CAD build for the part. Positions are in the model's coordinates, mm. A direction names the side the tool comes from. Coordinates: 2 decimals unless noted, no trailing zeros. Loops run counter-clockwise (first coordinate to the right, second up) from the corner with the lowest first, then second, coordinate; pieces in that order, holes last. Notation, with made-up numbers: (65, 58) -> (110, 58) arc R25 cw to (110, 77) -> close; hole circle Ø2 at (1.5, 68.5). An arc over 180 degrees is marked (long way). Write item = value, one per line. Start each with the question number.
(1) Tool access for faces 1 (the face through (2.958, -2.562, -32.586)), 2 (the face through (1.479, -11.495, -26.118)): list every direction of +Z, -Z, +X, -X, +Y, -Y with a clear straight run to the whole face (end or side of a thin tool).
(2) Pull direction Y, two halves, no side cores. Call faces 3 (the face through (2.96, -1.92, -10.54)), 4 (the face through (4.479, 12.156, -18.385)), 5 (the face through (4.48, -12.82, -17.36)), 6 (the face through (0, -3, -21)): +Y half, -Y half, draft (parallel to the pull), parting line (faces both ways), or undercut.
(3) Band-saw the part on C-C (x = 1.9). Write the cut outline in (y, z).
(4) Flat gauge pins, fed straight in: P1, Ø6, axis at y = -12.99, z = -21.36, coming from the +X side; P2, Ø3.5, axis at y = 12, z = -13.43, coming from the -X side; P3, Ø2, axis at x = 4, y = 0.5, coming from the -Z side. Where does each tip first touch, or does it go through?
(5) Band-saw the part on A-A (y = 12). Write the cut outline in (x, z), and give its area (3 significant figures).
(6) Drill centre lines: line 1 (Z direction, x = 3.95, y = 12); line 2 (Y direction, x = 5.55, z = -23.75); line 3 (Z direction, x = 1.25, y = -14.5). Where is each one in solid material? Low to high. Write a range as from..to.
(7) Band-saw the part on D-D (y = -10). Write the cut outline in (x, z), and give its area (3 significant figures).
(8) Band-saw the part on B-B (z = -24). Write the cut outline in (x, y), and give its area (3 significant figures).
```python
from build123d import *

# Parameters (mm, degrees)
SKETCH1_R           = 3.55
SKETCH1_R_2         = 1.5
SKETCH1_R_3         = 4
BOSS_EXTRUDE1_DEPTH = 6
SKETCH2_R           = 4.99
CUT_EXTRUDE1_DEPTH  = 3
SKETCH3_R           = 12.55
CUT_EXTRUDE2_DEPTH  = 3


with BuildPart() as part:
    # Sketch1 → Boss-Extrude1 (new body)
    with BuildSketch(Plane(origin=(0, 0, 0), x_dir=(0, 0, -1), z_dir=(1, 0, 0))):
        with BuildLine():
            Line((30.431712199, 18), (13.431712199, 18))
            ThreePointArc((13.431712199, 18), (8.728856289, 15.726009432), (7.590750373, 10.627715428))
            Line((7.590750373, 10.627715428), (13.570211844, -14.823132675))
            ThreePointArc((13.570211844, -14.823132675), (21.189386747, -20.991639419), (29.061992727, -15.150032042))
            Line((29.061992727, -15.150032042), (36.209586036, 10.382540903))
            ThreePointArc((36.209586036, 10.382540903), (35.212128216, 15.625965073), (30.431712199, 18))
        make_face()
        with Locations((21.931712199, 12)):
            Circle(SKETCH1_R, mode=Mode.SUBTRACT)
        with Locations((30.431712199, 12)):
            Circle(SKETCH1_R_2, mode=Mode.SUBTRACT)
        with Locations((13.431712199, 12)):
            Circle(SKETCH1_R_2, mode=Mode.SUBTRACT)
        with Locations((21.358160945, -12.993419913)):
            Circle(SKETCH1_R_3, mode=Mode.SUBTRACT)
    extrude(amount=BOSS_EXTRUDE1_DEPTH)

    # Sketch2 → Cut-Extrude1 (cut)
    with BuildSketch(Plane(origin=(0, 0, 0), x_dir=(0, 0, -1), z_dir=(1, 0, 0))):
        with Locations((21.358160945, -12.993419913)):
            Circle(SKETCH2_R)
    extrude(amount=CUT_EXTRUDE1_DEPTH, mode=Mode.SUBTRACT)

    # Sketch3 → Cut-Extrude2 (cut)
    with BuildSketch(Plane(origin=(0, 0, 0), x_dir=(0, 0, -1), z_dir=(1, 0, 0))):
        with Locations((21.931712199, 12)):
            Circle(SKETCH3_R)
    extrude(amount=CUT_EXTRUDE2_DEPTH, mode=Mode.SUBTRACT)


solid = part.part
```
Findings below:
q1.face_1 = -Z, +X, -X, -Y
q1.face_2 = -X
q2.face_3 = -Y half
q2.face_4 = undercut
q2.face_5 = undercut
q2.face_6 = draft
q3.outline = (-15.15, -29.06) -> (10.38, -36.21) arc R6 ccw to (17.25, -33.33) arc R12.55 cw (long way) to (17.25, -10.53) arc R6 ccw to (10.63, -7.59) -> (-14.82, -13.57) arc R8 ccw to start; hole circle Ø9.98 at (-12.99, -21.36)
q4.P1 = through
q4.P2 = 3
q4.P3 = -33.72
q5.outline = (0, -36.43) -> (6, -36.43) -> (6, -31.93) -> (3, -31.93) -> (3, -34.48) -> (0, -34.48) -> close; (0, -9.38) -> (3, -9.38) -> (3, -11.93) -> (6, -11.93) -> (6, -7.43) -> (0, -7.43) -> close; (3, -28.93) -> (6, -28.93) -> (6, -25.48) -> (3, -25.48) -> close; (3, -18.38) -> (6, -18.38) -> (6, -14.93) -> (3, -14.93) -> close
q5.area = 59.4 mm²
q6.line_1 = -36.43..-31.93, -28.93..-25.48, -18.38..-14.93, -11.93..-7.43
q6.line_2 = -20.63..-16.2, -9.79..8.95, 15.05..18
q6.line_3 = -29.24..-26.12, -16.6..-13.49
q7.outline = (0, -30.5) -> (6, -30.5) -> (6, -24.01) -> (3, -24.01) -> (3, -25.35) -> (0, -25.35) -> close; (0, -17.37) -> (3, -17.37) -> (3, -18.7) -> (6, -18.7) -> (6, -12.44) -> (0, -12.44) -> close
q7.area = 68.5 mm²
q8.outline = (0, -20.54) -> (6, -20.54) -> (6, -16) -> (3, -16) -> (3, -17.23) -> (0, -17.23) -> close; (0, -8.76) -> (3, -8.76) -> (3, -9.99) -> (6, -9.99) -> (6, 9.11) -> (3, 9.11) -> (3, -0.38) -> (0, -0.38) -> close; (3, 14.89) -> (6, 14.89) -> (6, 18) -> (3, 18) -> close
q8.area = 115 mm²
